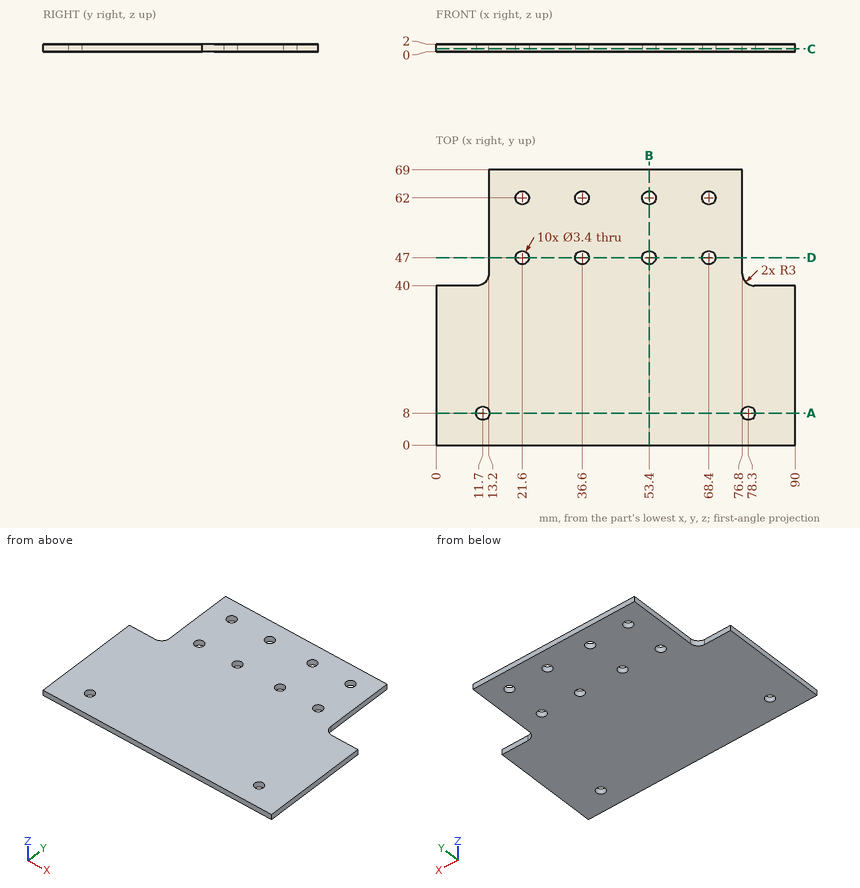
Print and shaded views of the part. All mm, measured from the part's lowest x, y and z. Coordinates: 2 decimals unless noted, no trailing zeros. Loops run counter-clockwise (first coordinate to the right, second up) from the corner with the lowest first, then second, coordinate; pieces in that order, holes last. Notation, with made-up numbers: M 44.25,49 L 85.25,49 A25 ccw 85.25,71 Z; hole C 71,58.5 d10. An arc over 180 degrees is marked long. Use a Markdown table: item, result. Add a question column.
Q1. Pin check, flat tips, straight feed: P1, Ø0.6, axis at y = 60.5, z = 1, coming from the -X side; P2, Ø1, axis at y = 54.5, z = 1, coming from the +X side; P3, Ø1, axis at x = 5, z = 0.5, coming from the +Y side. Stop position of each tip, or through.
Q2. Cut at D-D (y = 47). Write the cut outline in (x, z).
Q3. Cut at A-A (y = 8). Write the cut outline in (x, z).
Q4. Probe L1, parallel to Y at x = 53.4, z = 0.45; L2, parallel to X at y = 61, z = 1; L3, parallel to Y at x = 23, z = 0.5. List the from-to ranges inside material, lowest first.
Q5. Cut at B-B (x = 53.4). Write the cut outline in (y, z).
Q6. Cut at C-C (z = 0.8). Give the number of separate pieces and of enclosed holes in the cut face, and give its area (3 significant figures).
Worked out:
| question | item | result |
|---|---|---|
| 1 | P1 | stops at x = 13.2 |
| 1 | P2 | stops at x = 76.8 |
| 1 | P3 | stops at y = 40 |
| 2 | outline | M 13.2,0 L 19.9,0 L 19.9,2 L 13.2,2 Z; M 23.3,0 L 34.9,0 L 34.9,2 L 23.3,2 Z; M 38.3,0 L 51.7,0 L 51.7,2 L 38.3,2 Z; M 55.1,0 L 66.7,0 L 66.7,2 L 55.1,2 Z; M 70.1,0 L 76.8,0 L 76.8,2 L 70.1,2 Z |
| 3 | outline | M 0,0 L 10,0 L 10,2 L 0,2 Z; M 13.4,0 L 76.6,0 L 76.6,2 L 13.4,2 Z; M 80,0 L 90,0 L 90,2 L 80,2 Z |
| 4 | L1 | y = 0 to 45.3, 48.7 to 60.3, 63.7 to 69 |
| 4 | L2 | x = 13.2 to 20.23, 22.97 to 35.23, 37.97 to 52.03, 54.77 to 67.03, 69.77 to 76.8 |
| 4 | L3 | y = 0 to 46.04, 47.96 to 61.04, 62.96 to 69 |
| 5 | outline | M 0,0 L 45.3,0 L 45.3,2 L 0,2 Z; M 48.7,0 L 60.3,0 L 60.3,2 L 48.7,2 Z; M 63.7,0 L 69,0 L 69,2 L 63.7,2 Z |
| 6 | separate pieces | 1 |
| 6 | enclosed holes | 10 |
| 6 | area | 5,360 mm2 |
